The model under review builds one solid part; all positions refer to its coordinate system, in mm. Face numbers are marked on the shaded views. A direction names the side the tool comes from. Give positions to 0.01 mm unless a question says otherwise; leave off trailing zeros. Order: outer loops, then holes, each group sorted by start corner. A loop starts at its lowest first (then second) coordinate and runs counter-clockwise, first axis right, second up.
```python
from build123d import *

# Parameters (mm, degrees)
SKETCH_1_W           = 77
SKETCH_1_H           = 62.5
SKETCH_1_R           = 14
SKETCH_1_R_2         = 13
EXTRUDE_1_DEPTH      = 4
EXTRUDE_2_DEPTH      = 17
EXTRUDE_2_DEPTH_BACK = 13
FILLET_1_R           = 3
SKETCH_4_W           = 20
SKETCH_4_H           = 28.5
CUT_EXTRUDE_3_DEPTH  = 74
SKETCH_9_R           = 1.5
CUT_EXTRUDE_6_DEPTH  = 10
SKETCH_10_R          = 1.5
CUT_EXTRUDE_7_DEPTH  = 10
FILLET_2_R           = 5
CUT_EXTRUDE_8_DEPTH  = 10
FILLET_3_R           = 10
FILLET_4_R           = 3
SKETCH_13_R          = 14
SKETCH_13_R_2        = 12.5
EXTRUDE_3_DEPTH      = 1.5
SKETCH_14_R          = 11
CUT_EXTRUDE_9_DEPTH  = 10


with BuildPart() as part:
    # 草图1 → 凸台-拉伸1 (new body)
    with BuildSketch(Plane.XY):
        with Locations((10.5, 14.25)):
            Rectangle(SKETCH_1_W, SKETCH_1_H)
        Circle(SKETCH_1_R, mode=Mode.SUBTRACT)
        with Locations((26.381811917, 23)):
            Circle(SKETCH_1_R_2, mode=Mode.SUBTRACT)
    extrude(amount=EXTRUDE_1_DEPTH)

    # 草图1<3> → 凸台-拉伸2 (add, two sides: drawn at the far end of the back side and taken through both)
    with BuildSketch(Plane.XY.offset(-EXTRUDE_2_DEPTH_BACK)):
        Polygon((-52, 22.5), (-52, 26.5), (-28, 26.5), (-28, -2), (-52, -2), (-52, 2), (-32, 2), (-32, 22.5), align=None)
    extrude(amount=EXTRUDE_2_DEPTH + EXTRUDE_2_DEPTH_BACK)

    # 圆角1
    fillet_1_edges = [part.edges().sort_by_distance(p)[0] for p in [
        (-28, 12.25, 0),
        (-28, 12.25, 4),
    ]]
    fillet(fillet_1_edges, radius=FILLET_1_R)

    # 草图4 → 切除-拉伸3 (cut)
    with BuildSketch(Plane.XY.offset(17)):
        with Locations((-42, 12.25)):
            Rectangle(SKETCH_4_W, SKETCH_4_H)
    extrude(amount=-CUT_EXTRUDE_3_DEPTH, mode=Mode.SUBTRACT)

    # 草图9 → 切除-拉伸6 (cut)
    with BuildSketch(Plane.XY.offset(4)):
        with Locations((38.756180587, 35.374368671)):
            Circle(SKETCH_9_R)
        with Locations((38.756180587, 10.625631329)):
            Circle(SKETCH_9_R)
        with Locations((14.007443246, 10.625631329)):
            Circle(SKETCH_9_R)
        with Locations((14.007443246, 35.374368671)):
            Circle(SKETCH_9_R)
    extrude(amount=-CUT_EXTRUDE_6_DEPTH, mode=Mode.SUBTRACT)

    # 草图10 → 切除-拉伸7 (cut)
    with BuildSketch(Plane(origin=(-28, 0, 0), x_dir=(0, 0, -1), z_dir=(1, 0, 0))):
        with Locations((-13, 18.25)):
            Circle(SKETCH_10_R)
        with Locations((-13, 6.25)):
            Circle(SKETCH_10_R)
        with Locations((9, 18.25)):
            Circle(SKETCH_10_R)
        with Locations((9, 6.25)):
            Circle(SKETCH_10_R)
    extrude(amount=-CUT_EXTRUDE_7_DEPTH, mode=Mode.SUBTRACT)

    # 圆角2
    fillet_2_edges = [part.edges().sort_by_distance(p)[0] for p in [
        (-30, -2, 17),
        (-30, -2, -13),
        (-30, 26.5, 17),
        (-30, 26.5, -13),
    ]]
    fillet(fillet_2_edges, radius=FILLET_2_R)

    # 草图11 → 切除-拉伸8 (cut)
    with BuildSketch(Plane.XY.offset(4)):
        Polygon((-28, 29.5), (-28, 45.5), (-12, 45.5), align=None)
        Polygon((19, -17), (49, 13), (49, -17), align=None)
    extrude(amount=-CUT_EXTRUDE_8_DEPTH, mode=Mode.SUBTRACT)

    # 圆角3
    fillet_3_edges = [part.edges().sort_by_distance(p)[0] for p in [
        (-28, -17, 2),
        (49, 45.5, 2),
    ]]
    fillet(fillet_3_edges, radius=FILLET_3_R)

    # 圆角4
    fillet_4_edges = [part.edges().sort_by_distance(p)[0] for p in [
        (-28, -2, 2),
        (-28, 26.5, 2),
    ]]
    fillet(fillet_4_edges, radius=FILLET_4_R - 0.0001)  # a hair under: the kernel refuses the full size

    # 草图13 → 凸台-拉伸3 (add)
    with BuildSketch(Plane(origin=(0, 0, 0), x_dir=(-1, 0, 0), z_dir=(0, 0, -1))):
        Circle(SKETCH_13_R)
        Circle(SKETCH_13_R_2, mode=Mode.SUBTRACT)
    extrude(amount=-EXTRUDE_3_DEPTH)

    # 草图14 → 切除-拉伸9 (cut)
    with BuildSketch(Plane.XY.offset(4)):
        with Locations((-5, 29.5)):
            Circle(SKETCH_14_R)
    extrude(amount=-CUT_EXTRUDE_9_DEPTH, mode=Mode.SUBTRACT)


solid = part.part
```
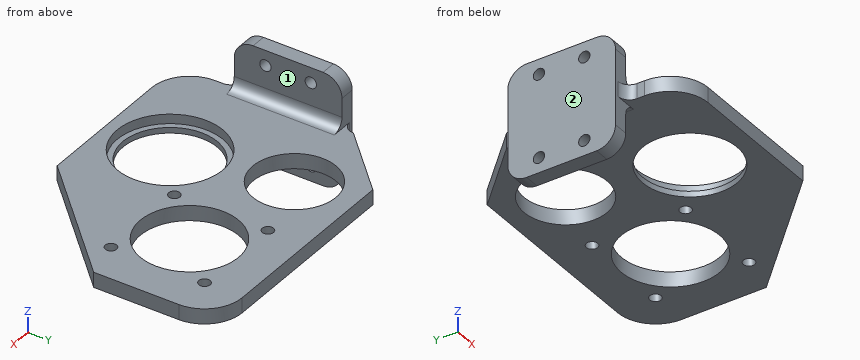
1. For the marked faces 1 and 2, list the 3-axis set-ups (+Z, -Z, +X, -X, +Y, -Y) from which the entire face can be reached by the end or side of a thin tool; tool diameter is ignored.
2. Take a section at D-D (y = 23). Write out the cut boundary in (x, z).
3. Insertion check: pin 1 (5 mm diameter, centred on y = 9, z = 12.5, fed in from +X); pin 2 (2.5 mm diameter, centred on y = 18.25, z = 13, fed in from -X); pin 3 (5 mm diameter, centred on x = 33, z = 0.5, fed in from -Y); pin 4 (2 mm diameter, centred on y = -5, z = -0.5, fed in from -X). Each pin has a flat end and moves straight along its axis. Give the tip position at first contact, or say it passes through.
4. Take a section at C-C (x = -5). Write out the cut boundary in (y, z).
5. Take a section at A-A (z = 13). Write out the cut boundary in (x, y).
6. Take a section at B-B (y = 15.5). Write out the cut boundary in (x, z).
7. To check wall thickness, follow line 1 (Y direction, x = -5, z = 1.4); line 2 (Z direction, x = 23, y = -3.5); line 3 (Y direction, x = 0, z = 3.1). State the ranges of each line that lie inside material, in increasing order.
Answer:
1. face 1: +Z, +X, +Y, -Y
1. face 2: +Z, -Z, -X, +Y, -Y
2. outline: (-32, -12.77) - (-28, -12.77) - (-28, -3) arc R3 cw to (-25, 0) - (-13.87, 0) - (-13.87, 4) - (-25, 4) arc R3 cw to (-28, 7) - (-28, 16.77) - (-32, 16.77) - close; (3.87, 0) - (13.38, 0) - (13.38, 4) - (3.87, 4) - close; (39.38, 0) - (49, 0) - (49, 4) - (39.38, 4) - close
3. pin 1: stops at x = -28
3. pin 2: passes through
3. pin 3: stops at y = -5.5
3. pin 4: stops at x = -28.13
4. outline: (-17, 0) - (-11.46, 0) - (-11.46, 1.5) - (-13.08, 1.5) - (-13.08, 4) - (-17, 4) - close; (11.46, 0) - (18.5, 0) - (18.5, 4) - (13.08, 4) - (13.08, 1.5) - (11.46, 1.5) - close; (40.5, 0) - (45.5, 0) - (45.5, 4) - (40.5, 4) - close
5. outline: (-32, -1.9) - (-28, -1.9) - (-28, 4.75) - (-32, 4.75) - close; (-32, 7.75) - (-28, 7.75) - (-28, 16.75) - (-32, 16.75) - close; (-32, 19.75) - (-28, 19.75) - (-28, 26.4) - (-32, 26.4) - close
6. outline: (-32, -13) - (-28, -13) - (-28, -3) arc R3 cw to (-25, 0) - (15.76, 0) - (15.76, 4) - (-25, 4) arc R3 cw to (-28, 7) - (-28, 17) - (-32, 17) - close; (37, 0) - (49, 0) - (49, 4) - (37, 4) - close
7. line 1: y = -17 to -11.46, 11.46 to 18.5, 40.5 to 45.5
7. line 2: z = 0 to 4
7. line 3: y = -17 to -14, 14 to 19.7, 39.3 to 45.5
